Here's how the part is built. I have some questions about the finished solid (model axes, mm). Face numbers are marked on the shaded views. Round coordinates to 2 decimals unless told otherwise and drop trailing zeros. Loops run counter-clockwise (first coordinate to the right, second up) from the corner with the lowest first, then second, coordinate; pieces in that order, holes last. Notation, with made-up numbers: M 45,-24 L 59,-24 A27 cw 59,-1 Z; hole C 36,53 d1. An arc over 180 degrees is marked long. Answer as a JSON object with one key per item and string values.
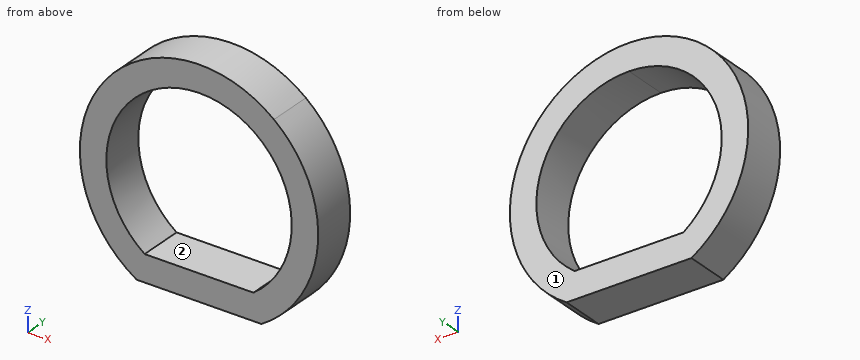
from build123d import *

# Parameters (mm, degrees)
BOSS_EXTRU_2_DEPTH = 5


with BuildPart() as part:
    # Esquisse2 → Boss.-Extru.2 (new body)
    with BuildSketch(Plane(origin=(0, 0, 0), x_dir=(1, 0, 0), z_dir=(0, 1, 0))):
        with BuildLine():
            ThreePointArc((-19.751463333, 34.064312188), (-23.703099364, 14.770083553), (-4.195114147, 12.064312188))
            ThreePointArc((-4.195114147, 12.064312188), (0.791798064, 23.430337591), (-5.609327709, 34.064312188))
            Line((-5.609327709, 34.064312188), (-19.751463333, 34.064312188))
        make_face()
        with BuildLine():
            Line((-18.844809524, 31.064312188), (-6.515981518, 31.064312188))
            ThreePointArc((-6.515981518, 31.064312188), (-2.692903343, 19.323941838), (-12.680395521, 12.064312188))
            ThreePointArc((-12.680395521, 12.064312188), (-22.667887699, 19.323941838), (-18.844809524, 31.064312188))
        make_face(mode=Mode.SUBTRACT)
    extrude(amount=BOSS_EXTRU_2_DEPTH)


solid = part.part
Item 1: I want a section at C-C on y = 3. List the corners of the cut face in (x, z) for me, plus the area to 3 significant figures.
Solution:
{"outline": "M -19.75,-34.06 L -5.61,-34.06 A13.5 ccw long Z; hole M -18.84,-31.06 L -6.52,-31.06 A10.5 ccw long Z", "area": "224 mm2"}
Item 2: I want a section at D-D on z = -11. List the corners of the cut face in (x, y) for me (3 decimals), plus the area to 3 significant figures.
Solution:
{"outline": "M -19.646,0 L -5.715,0 L -5.715,5 L -19.646,5 Z", "area": "69.7 mm2"}
Item 3: For P1, Ø8, axis at x = -18.5, z = -25, coming from the -Y side; P2, Ø1.5, axis at y = 2.5, z = -12.5, coming from the -X side; P3, Ø1.5, axis at x = -22.5, y = 1.5, coming from the +Z side; P4, Ø1, axis at x = -21, y = 3.5, coming from the -Z side, each with a flat end and sliding along its axis, tell me the tip position at first contact or that it passes through.
Solution:
{"P1": "passes through", "P2": "stops at x = -22.45", "P3": "stops at z = -12.56", "P4": "stops at z = -33.57"}
Item 4: I want a section at B-B on x = -14.5. List the corners of the cut face in (y, z) for me.
Solution:
{"outline": "M 0,-34.06 L 5,-34.06 L 5,-31.06 L 0,-31.06 Z; M 0,-12.22 L 5,-12.22 L 5,-9.19 L 0,-9.19 Z"}
Item 5: We'd pull the mould along X, two halves only. Please class the marked faces 1 and 2: +X half, -X half, draft (parallel to the pull), parting line (faces both ways), or undercut.
Solution:
{"face 1": "draft", "face 2": "undercut"}
Item 6: If I drill on L1, parallel to Z at x = -13, y = 1; L2, parallel to X at y = 3.9, z = -31; L3, parallel to X at y = 1.15, z = -25.5, over which ranges is the centre line in solid material (lowest first)? Write a range as from..to.
Solution:
{"L1": "z = -34.06..-31.06, -12.07..-9.07", "L2": "x = -23.22..-18.93, -6.43..-2.14", "L3": "x = -25.86..-22.76, -2.6..0.5"}
Item 7: I want a section at A-A on z = -23.75. List the corners of the cut face in (x, y) for me.
Solution:
{"outline": "M -26.13,0 L -23.11,0 L -23.11,5 L -26.13,5 Z; M -2.25,0 L 0.77,0 L 0.77,5 L -2.25,5 Z"}
